from build123d import *

# Parameters (mm, degrees)
SKETCH1_R           = 1.5
BOSS_EXTRUDE1_DEPTH = 10
CHAMFER1_SIZE       = 0.25
CHAMFER1_SIZE2      = 0.144337567
SKETCH2_R           = 3
BOSS_EXTRUDE2_DEPTH = 2.5
FILLET1_R           = 1
CUT_EXTRUDE1_DEPTH  = 2


with BuildPart() as part:
    # Sketch1 → Boss-Extrude1 (new body)
    with BuildSketch(Plane(origin=(0, 0, 0), x_dir=(1, 0, 0), z_dir=(0, 1, 0))):
        with Locations(Location((0, 0, 0), (0, 0, 270))):
            Circle(SKETCH1_R)
    extrude(amount=BOSS_EXTRUDE1_DEPTH)

    # Chamfer1
    chamfer1_edges = [part.edges().sort_by_distance(p)[0] for p in [
        (0, 10, -1.5),
    ]]
    chamfer1_side = [part.faces().sort_by_distance(p)[0] for p in [
        (0, 5, -1.5),
    ]]
    chamfer(chamfer1_edges, length=CHAMFER1_SIZE, length2=CHAMFER1_SIZE2, reference=chamfer1_side[0])

    # Sketch2 → Boss-Extrude2 (add)
    with BuildSketch(Plane(origin=(0, 0, 0), x_dir=(-1, 0, 0), z_dir=(0, -1, 0))):
        with Locations(Location((0, 0, 0), (0, 0, 90))):
            Circle(SKETCH2_R)
    extrude(amount=BOSS_EXTRUDE2_DEPTH)

    # Fillet1
    fillet1_edges = [part.edges().sort_by_distance(p)[0] for p in [
        (0, -2.5, 3),
    ]]
    fillet(fillet1_edges, radius=FILLET1_R)

    # Sketch3 → Cut-Extrude1 (cut)
    with BuildSketch(Plane(origin=(0, -2.5, 0), x_dir=(-1, 0, 0), z_dir=(0, -1, 0))):
        Polygon((1.58771324, 0), (0.79385662, 1.375), (-0.79385662, 1.375), (-1.58771324, 0), (-0.79385662, -1.375), (0.79385662, -1.375), align=None)
    extrude(amount=-CUT_EXTRUDE1_DEPTH, mode=Mode.SUBTRACT)


solid = part.part
Here's how the part is built. I have some questions about the finished solid (model axes, mm). A direction names the side the tool comes from. Coordinates: 2 decimals unless noted, no trailing zeros. Write each loop counter-clockwise with the first axis right and the second up, starting at its lowest first coordinate (ties: lowest second). Pieces come first, ordered by that corner, then holes.
1) Thinking about a two-plate mould opening in X: for faces 1 (the face through (0, 10, 0)), 2 (the face through (1.196, -1.514, 0.678)), 3 (the face through (0.45, 4.81, 1.43)), which applies, +X half, -X half, draft (parallel to the pull), parting line (faces both ways), or undercut?
Filled in:
face 1: draft
face 2: undercut
face 3: parting line
2) If we section it at A-A (x = 0): List the corners of the cut face in (y, z) for me (3 decimals).
Filled in:
outline: (-2.5, -2) arc R1 ccw to (-1.5, -3) - (0, -3) - (0, -1.5) - (9.75, -1.5) - (10, -1.356) - (10, 1.356) - (9.75, 1.5) - (0, 1.5) - (0, 3) - (-1.5, 3) arc R1 ccw to (-2.5, 2) - (-2.5, 1.375) - (-0.5, 1.375) - (-0.5, -1.375) - (-2.5, -1.375) - close
3) Which directions (+Z, -Z, +X, -X, +Y, -Y) give clear straight access to the entire face, cutting with the end or side of a thin tool? Please do faces 4 (the face through (-1.3, 0, -1.3)), 5 (the face through (-1.3, -2.5, -0.9)), 6 (the face through (0, -2, -1.375)).
Filled in:
face 4: +Y
face 5: +Z, -Z, +X, -X, -Y
face 6: -Y
4) If I drill on line 1 (Y direction, x = 1, z = 0.35); line 2 (Y direction, x = -1.25, z = -1.2); line 3 (X direction, y = -2, z = 0.5), over which ranges is the centre line in solid material (lowest first)?
Filled in:
line 1: y = -0.5 to 10
line 2: y = -2.5 to 0
line 3: x = -2.82 to -1.3, 1.3 to 2.82
5) If we section it at B-B (y = 5.25): List the corners of the cut face in (x, z) for me.
Filled in:
outline: circle Ø3 at (0, 0)
6) I'm going to push flat-ended pins straight in: pin 1 (3 mm diameter, centred on y = 4, z = 0, fed in from -X); pin 2 (1.4 mm diameter, centred on x = -0.5, z = 0, fed in from -Y); pin 3 (3 mm diameter, centred on x = 0.5, y = 0.5, fed in from +Z); pin 4 (0.5 mm diameter, centred on x = -0.5, y = -2, fed in from -Z). Where does each tip first touch, or does it pass through?
Filled in:
pin 1: stops at x = -1.5
pin 2: stops at y = -0.5
pin 3: stops at z = 3
pin 4: stops at z = -2.94
